Can you work these out from the drawing? Everything is in mm from the part's minimum corner. A direction names the side the tool comes from. Coordinates: 2 decimals unless noted, no trailing zeros. Loops run counter-clockwise (first coordinate to the right, second up) from the corner with the lowest first, then second, coordinate; pieces in that order, holes last.
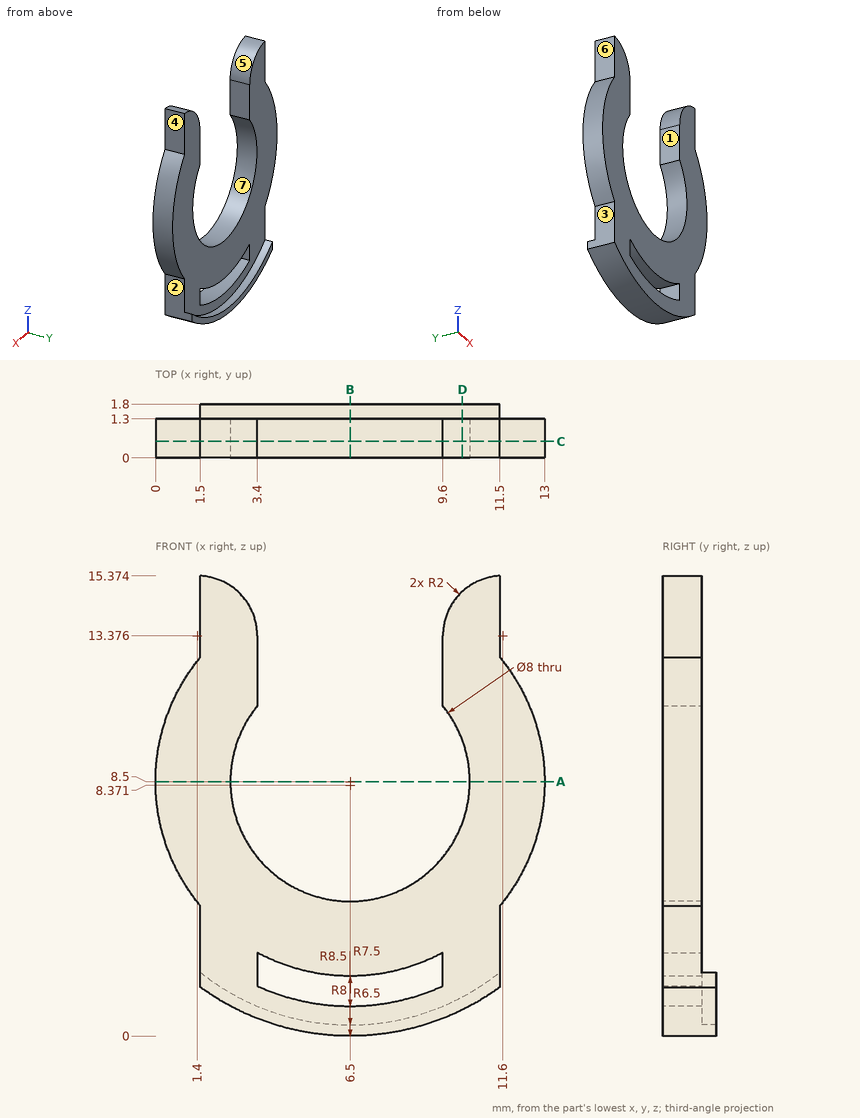
Item 1: We'd pull the mould along X, two halves only. Please class the marked faces 1, 2 and 3: +X half, -X half, draft (parallel to the pull), parting line (faces both ways), or undercut.
Results are:
face 1: undercut
face 2: +X half
face 3: -X half
Item 2: I'm going to push flat-ended pins straight in: P1, Ø1, axis at x = 4, z = 3.5, coming from the +Y side; P2, Ø0.6, axis at y = 0.5, z = 14, coming from the +X side; P3, Ø0.5, axis at y = 0.5, z = 2.5, coming from the -X side. Where does each tip first touch, or does it pass through?
Results are:
P1: stops at y = 1.3
P2: stops at x = 11.5
P3: stops at x = 1.5
Item 3: Suppose I cut it at D-D, the plane x = 10.25. Please give me the cut outline in (y, z) (1 decimal).
Results are:
outline: (0, 0.9) - (1.8, 0.9) - (1.8, 1.3) - (1.3, 1.3) - (1.3, 7.1) - (0, 7.1) - close; (0, 9.9) - (1.3, 9.9) - (1.3, 14.9) - (0, 14.9) - close
Item 4: On a 3-axis mill with a long thin cutter (end or side, diameter ignored), from which of +Z, -Z, +X, -X, +Y, -Y can I reach the whole of each face in a straight line? I mean the marked faces 4, 5, 6 and 7. Say none if no direction works.
Results are:
face 4: +Z, +X, +Y, -Y
face 5: +Z, +Y, -Y
face 6: +Z, -X, +Y, -Y
face 7: +Y, -Y
Item 5: I need wall thicknesses on line 1 along X through (y, z) = (0.9, 8.5); line 2 along Z through (x, y) = (6.75, 1.65) (1 decimal); line 3 along X through (y, z) = (0.4, 5) (1 decimal). Which ranges of each line are inside material? Lowest first, please.
Results are:
line 1: x = 0 to 2.5, 10.5 to 13
line 2: z = 0 to 0.4
line 3: x = 1 to 4.6, 8.4 to 12
Item 6: Suppose I cut it at A-A, the plane z = 8.5. Please give me the cut outline in (x, y).
Results are:
outline: (0, 0) - (2.5, 0) - (2.5, 1.3) - (0, 1.3) - close; (10.5, 0) - (13, 0) - (13, 1.3) - (10.5, 1.3) - close
Item 7: Suppose I cut it at C-C, the plane y = 0.55. Please give me the cut outline in (x, z).
Results are:
outline: (1.5, 1.63) arc R8.5 ccw to (11.5, 1.63) - (11.5, 4.35) arc R6.5 ccw to (11.5, 12.65) - (11.5, 15.37) arc R2 ccw to (9.6, 13.38) - (9.6, 11.03) arc R4 cw (long way) to (3.4, 11.03) - (3.4, 13.38) arc R2 ccw to (1.5, 15.37) - (1.5, 12.65) arc R6.5 ccw to (1.5, 4.35) - close; hole (3.4, 1.67) arc R7.5 ccw to (9.6, 1.67) - (9.6, 2.79) arc R6.5 cw to (3.4, 2.79) - close
Item 8: Suppose I cut it at B-B, the plane x = 6.5. Please give me the cut outline in (y, z).
Results are:
outline: (0, 0) - (1.8, 0) - (1.8, 0.37) - (1.3, 0.37) - (1.3, 1) - (0, 1) - close; (0, 2) - (1.3, 2) - (1.3, 4.5) - (0, 4.5) - close
